Geometry: final body of the model. Coordinates: model frame, mm. Face numbers are marked on the shaded views. A direction names the side the tool comes from. Round coordinates to 2 decimals unless told otherwise and drop trailing zeros. Loops run counter-clockwise (first coordinate to the right, second up) from the corner with the lowest first, then second, coordinate; pieces in that order, holes last. Notation, with made-up numbers: (37.5, 45) - (63.5, 45) arc R27 cw to (63.5, 78) - close; hole circle Ø6 at (49, 89). An arc over 180 degrees is marked (long way). Answer as CSV lines item,"result".
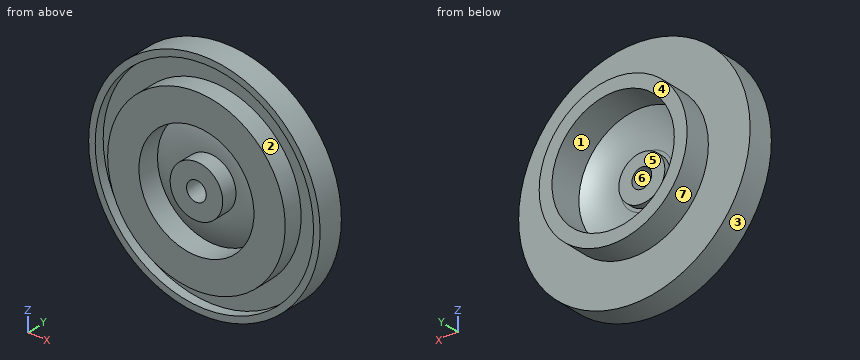
from build123d import *

# Parameters (mm, degrees)
SKETCH2_R          = 1.5
CUT_EXTRUDE1_DEPTH = 10


with BuildPart() as part:
    # Sketch1 → Revolve1 (revolve)
    with BuildSketch(Plane.XY):
        with BuildLine():
            Line((-17.6, 1.5), (-17.6, 5.5))
            Line((-17.6, 5.5), (-11.25, 5.5))
            Line((-11.25, 5.5), (-11.25, 9.5))
            Line((-11.25, 9.5), (-9.3, 9.5))
            Line((-9.3, 9.5), (-9.3, 4.435928697))
            ThreePointArc((-9.3, 4.435928697), (-6.732887918, 3.439124969), (-4, 3.1))
            Line((-4, 3.1), (-3.5, 3.1))
            Line((-3.5, 3.1), (-3.5, 4.1))
            Line((-3.5, 4.1), (0, 4.1))
            Line((0, 4.1), (0, 0))
            Line((0, 0), (-4, 0))
            Line((-4, 0), (-4, 2.5))
            ThreePointArc((-4, 2.5), (-6.42706098, 2.752710346), (-8.75, 3.5))
            Line((-8.75, 3.5), (-8.75, 0))
            Line((-8.75, 0), (-13.5, 0))
            Line((-13.5, 0), (-13.5, 3))
            Line((-13.5, 3), (-16.6, 3))
            Line((-16.6, 3), (-16.6, 1.5))
            Line((-16.6, 1.5), (-17.6, 1.5))
        make_face()
    revolve(axis=Axis((0, 0, 0), (0, 1, 0)))

    # Sketch2 → Cut-Extrude1 (cut)
    with BuildSketch(Plane(origin=(0, 4.1, 0), x_dir=(1, 0, 0), z_dir=(0, 1, 0))):
        Circle(SKETCH2_R)
    extrude(amount=-CUT_EXTRUDE1_DEPTH, mode=Mode.SUBTRACT)


solid = part.part
(1) Material intervals for line 1 along Z through (x, y) = (0, 1); line 2 along Z through (x, y) = (0, 1.95); line 3 along Z through (x, y) = (0, 5.9), sorted ascending.
Findings below:
line 1,"-13.5 to -8.75, -4 to -1.5, 1.5 to 4, 8.75 to 13.5"
line 2,"-17.6 to -16.6, -13.5 to -8.75, -4 to -1.5, 1.5 to 4, 8.75 to 13.5, 16.6 to 17.6"
line 3,"-11.25 to -9.3, 9.3 to 11.25"
(2) Access query for the marked faces 1, 2 and 3. Directions: +Z, -Z, +X, -X, +Y, -Y. A direction counts if a zero-diameter tool reaches every point of the face in a straight line with its end or side. Return the directions, or none.
Findings below:
face 1,"+Y"
face 2,"-Y"
face 3,"+Y, -Y"
(3) Section C-C (x = -13). Output: boundary loops of the cut face in (y, z).
Findings below:
outline,"(0, -3.64) - (3, -3.64) - (3, -10.32) - (1.5, -10.32) - (1.5, -11.86) - (5.5, -11.86) - (5.5, 11.86) - (1.5, 11.86) - (1.5, 10.32) - (3, 10.32) - (3, 3.64) - (0, 3.64) - close"
(4) Section A-A (y = 7.25). Output: boundary loops of the cut face in (x, z).
Findings below:
outline,"circle Ø22.5 at (0, 0); hole circle Ø18.6 at (0, 0)"
(5) Draft query along Z for the marked faces 4, 5, 6 and 7. Return one class per face: pulls with the +Z half, pulls with the -Z half, needs draft (parallel to the pull), parting line crosses it, or undercut.
Findings below:
face 4,"needs draft"
face 5,"undercut"
face 6,"undercut"
face 7,"parting line crosses it"
(6) Section B-B (z = 12). Output: boundary loops of the cut face in (x, y).
Findings below:
outline,"(-12.87, 1.5) - (-11.47, 1.5) - (-11.47, 3) - (-6.18, 3) - (-6.18, 0) - (6.18, 0) - (6.18, 3) - (11.47, 3) - (11.47, 1.5) - (12.87, 1.5) - (12.87, 5.5) - (-12.87, 5.5) - close"
(7) Pin query (flat end, axial travel): P1, Ø1.5, axis at x = 13.5, y = 8.5, coming from the -Z side; P2, Ø4, axis at x = 3, y = 1.5, coming from the -Z side; P3, Ø5, axis at x = -4, y = 2, coming from the +Z side; P4, Ø2.5, axis at x = 0, z = -1, coming from the +Y side. Return the tip coordinate at first contact, or that it passes through.
Findings below:
P1,"through"
P2,"z = -17.57"
P3,"z = 17.54"
P4,"y = 4.1"
